Design review of the part built by this model. Coordinates are the model's own, in mm. Face numbers are marked on the shaded views. A direction names the side the tool comes from. Give positions to 0.01 mm unless a question says otherwise; leave off trailing zeros. Loops run counter-clockwise (first coordinate to the right, second up) from the corner with the lowest first, then second, coordinate; pieces in that order, holes last. Notation, with made-up numbers: (83, 84) - (134, 84) arc R16 ccw to (134, 91) - close; hole circle Ø1 at (10.25, 58). An arc over 180 degrees is marked (long way). Write each question's results on one line, items separated by ' | '.
```python
from build123d import *

# Parameters (mm, degrees)
F0_W     = 45
F0_H     = 63
F1_DEPTH = 24
F3_DEPTH = 21
F4_R     = 2.5
F5_DEPTH = 3


with BuildPart() as f1:
    # F0 (on Top) → F1 (new body)
    with BuildSketch(Plane.XY):
        Rectangle(F0_W, F0_H)
    extrude(amount=F1_DEPTH)

    # F2 (on face) → F3 (cut)
    with BuildSketch(Plane.XY.offset(24)):
        with BuildLine():
            Line((5, 31.5), (-5, 31.5))
            Line((-5, 31.5), (-5, 24))
            ThreePointArc((-5, 24), (0, 19), (5, 24))
            Line((5, 24), (5, 31.5))
        make_face()
        with BuildLine():
            Line((-5, -24), (-5, -31.5))
            Line((-5, -31.5), (5, -31.5))
            Line((5, -31.5), (5, -24))
            ThreePointArc((5, -24), (0, -19), (-5, -24))
        make_face()
    extrude(amount=-F3_DEPTH, mode=Mode.SUBTRACT)

    # F4 (on face) → F5 (cut, through all)
    with BuildSketch(Plane.XY.offset(3)):
        with Locations((0, 24)):
            Circle(F4_R)
        with BuildLine():
            Line((2.5, -26), (2.5, -22))
            ThreePointArc((2.5, -22), (0, -19.5), (-2.5, -22))
            Line((-2.5, -22), (-2.5, -26))
            ThreePointArc((-2.5, -26), (0, -28.5), (2.5, -26))
        make_face()
    extrude(amount=-F5_DEPTH, mode=Mode.SUBTRACT)


solid = f1.part
```
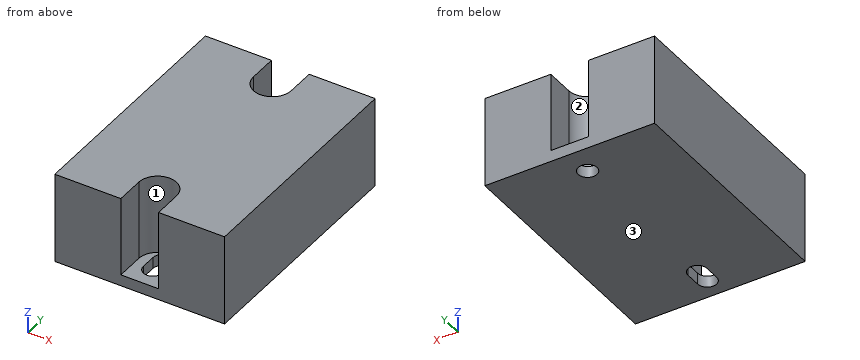
Item 1: Clearance check with a flat-ended pin moving along its axis: P1, Ø5, axis at x = 1, y = -25.5, coming from the +Z side. State where the tip first meets the part, or that it passes through.
Output values:
P1: stops at z = 3
Item 2: Wall thickness on probe 1 along Y at (x, z) = (0, 1.65); probe 2 along X at (y, z) = (-27, 15.25); probe 3 along X at (y, z) = (-26.5, 1.75): over which ranges is each line inside the solid? List them lowest first.
Output values:
probe 1: y = -31.5 to -28.5, -19.5 to 21.5, 26.5 to 31.5 | probe 2: x = -22.5 to -5, 5 to 22.5 | probe 3: x = -22.5 to -2.45, 2.45 to 22.5
Item 3: We need section A-A on z = 2.25. Give the boundary of the cut face in (x, y), then the cut area to 3 significant figures.
Output values:
outline: (-22.5, -31.5) - (22.5, -31.5) - (22.5, 31.5) - (-22.5, 31.5) - close; hole (-2.5, -26) arc R2.5 ccw to (2.5, -26) - (2.5, -22) arc R2.5 ccw to (-2.5, -22) - close; hole circle Ø5 at (0, 24) | area: 2,780 mm²
Item 4: We need section C-C on z = 19.75. Give the boundary of the cut face in (x, y).
Output values:
outline: (-22.5, -31.5) - (-5, -31.5) - (-5, -24) arc R5 cw to (5, -24) - (5, -31.5) - (22.5, -31.5) - (22.5, 31.5) - (5, 31.5) - (5, 24) arc R5 cw to (-5, 24) - (-5, 31.5) - (-22.5, 31.5) - close
Item 5: Tool access review of the marked faces 1, 2 and 3: name each direction out of +Z, -Z, +X, -X, +Y, -Y from which nothing blocks a thin tool from reaching the whole face with its end or side.
Output values:
face 1: +Z, -Y | face 2: +Z, +Y | face 3: -Z, +X, -X, +Y, -Y
Item 6: We need section B-B on x = 0. Give the boundary of the cut face in (y, z).
Output values:
outline: (-31.5, 0) - (-28.5, 0) - (-28.5, 3) - (-31.5, 3) - close; (-19.5, 0) - (21.5, 0) - (21.5, 3) - (19, 3) - (19, 24) - (-19, 24) - (-19, 3) - (-19.5, 3) - close; (26.5, 0) - (31.5, 0) - (31.5, 3) - (26.5, 3) - close
